from build123d import *

# Parameters (mm, degrees)
SKETCH1_R           = 8.75
BOSS_EXTRUDE1_DEPTH = 15
SKETCH2_R           = 1.9
CUT_EXTRUDE1_DEPTH  = 20
SKETCH3_R           = 1.9
CUT_EXTRUDE2_DEPTH  = 10
SKETCH4_W           = 24.600517232
SKETCH4_H           = 3.517349106
SKETCH4_W_2         = 3.50600932
SKETCH4_W_3         = 2.117023419
CUT_EXTRUDE3_DEPTH  = 129
SKETCH5_W           = 14.928012143
SKETCH5_H           = 3.517349106
CUT_EXTRUDE4_DEPTH  = 39.5


with BuildPart() as part:
    # Sketch1 → Boss-Extrude1 (new body)
    with BuildSketch(Plane(origin=(0, 0, 0), x_dir=(1, 0, 0), z_dir=(0, 1, 0))):
        with BuildLine():
            Line((7.55, -6.557247898), (7.55, -9.961620247))
            Line((7.55, -9.961620247), (14.289149279, -9.92724627))
            Line((14.289149279, -9.92724627), (14.289149279, -7.931016803))
            Line((14.289149279, -7.931016803), (8.967681349, -7.931016803))
            Line((8.967681349, -7.931016803), (8.967681349, -4.425007483))
            ThreePointArc((8.967681349, -4.425007483), (9.738501258, -2.271914007), (10, 0))
            ThreePointArc((10, 0), (-0.861319558, 10.861319558), (-11.722639117, 0))
            Line((-11.722639117, 0), (-11.722639117, -16.005864092))
            Line((-11.722639117, -16.005864092), (-10, -16.005864092))
            Line((-10, -16.005864092), (-10, 0))
            ThreePointArc((-10, 0), (-3.5, -9.367496998), (7.55, -6.557247898))
        make_face()
        with Locations(Location((0, 0, 0), (0, 0, 270))):
            Circle(SKETCH1_R, mode=Mode.SUBTRACT)
    extrude(amount=-BOSS_EXTRUDE1_DEPTH)

    # Sketch2 → Cut-Extrude1 (cut, symmetric)
    with BuildSketch(Plane.ZY.offset(10.823854245)):
        with Locations(Location((12.870484291, -12, 0), (0, 0, 180))):
            Circle(SKETCH2_R)
        with Locations(Location((12.870484291, -3, 0), (0, 0, 180))):
            Circle(SKETCH2_R)
    extrude(amount=CUT_EXTRUDE1_DEPTH, both=True, mode=Mode.SUBTRACT)

    # Sketch3 → Cut-Extrude2 (cut)
    with BuildSketch(Plane(origin=(0, 0, 7.931016803), x_dir=(-1, 0, 0), z_dir=(0, 0, -1))):
        with Locations((-11.586638558, -12.051447382)):
            Circle(SKETCH3_R)
        with Locations((-11.586638558, -3.07185738)):
            Circle(SKETCH3_R)
    extrude(amount=-CUT_EXTRUDE2_DEPTH, mode=Mode.SUBTRACT)

    # Sketch4 → Cut-Extrude3 (cut)
    with BuildSketch(Plane(origin=(8.967681349, 0, 0), x_dir=(0, 0, -1), z_dir=(1, 0, 0))):
        with Locations((7.875251133, -7.5)):
            Rectangle(SKETCH4_W, SKETCH4_H)
        with Locations((-6.178012143, -7.5)):
            Rectangle(SKETCH4_W_2, SKETCH4_H)
        with Locations((-8.989528513, -7.5)):
            Rectangle(SKETCH4_W_3, SKETCH4_H)
    extrude(amount=-CUT_EXTRUDE3_DEPTH, mode=Mode.SUBTRACT)

    # Sketch5 → Cut-Extrude4 (cut, symmetric)
    with BuildSketch(Plane(origin=(-10, 0, 0), x_dir=(0, 0, -1), z_dir=(1, 0, 0))):
        with Locations((1.285993928, -7.5)):
            Rectangle(SKETCH5_W, SKETCH5_H)
    extrude(amount=CUT_EXTRUDE4_DEPTH, both=True, mode=Mode.SUBTRACT)


solid = part.part
Read the model definition and answer for the solid it produces. Units are mm, in the model's axes. A direction names the side the tool comes from. Round coordinates to 2 decimals unless told otherwise and drop trailing zeros. Order: outer loops, then holes, each group sorted by start corner. A loop starts at its lowest first (then second) coordinate and runs counter-clockwise, first axis right, second up. Notation, with made-up numbers: (45, -7) - (60, -7) arc R21 ccw to (60, 11) - close; hole circle Ø7 at (52, 24.25). An arc over 180 degrees is marked (long way). Use one line per item in the form item = value. Start each with the question number.
(1) Flat-ended cylindrical pins translate along their axes: pin 1 Ø3.5 at (y, z) = (-12, 12.87) entering from +X; pin 2 Ø0.9 at (x, y) = (-11, -7.5) entering from -Z; pin 3 Ø6 at (x, y) = (-7.5, -8) entering from -Z; pin 4 Ø2 at (x, y) = (2, -6.5) entering from +Z. Find the tip coordinate at first contact, or state that the pin passes through.
(2) For faces 5 (the face through (7.55, -12, 8)), 6 (the face through (-9, -9.259, 0)), 7 (the face through (12, -7, 7.931)), 8 (the face through (-11, -8, 10.048)), determine the directions among +Z, -Z, +X, -X, +Y, -Y from which every point of the face is accessible in a straight line to the end or side of a thin tool.
(3) Determine the mould class of faces 1 (the face through (8.968, -3, 6)), 2 (the face through (-0.62, -2.83, -10.86)), 3 (the face through (-3.659, -2.83, 9.307)), 4 (the face through (-10.87, -3.08, 14.77)) for opening direction X: +X half, -X half, draft (parallel to the pull), parting line (faces both ways), or undercut.
(4) The part is cut by section A-A (y = -6.5). Give the vertices of the cut face in (x, z), then the cut area to 3 significant figures.
(5) The part is cut by section B-B (y = -1.75). Give the vertices of the cut face in (x, z) (3 decimals).
(6) The part is cut by section C-C (z = -3.5). Give the vertices of the cut face in (x, y), then the cut area to 3 significant figures.
(7) Find the intervals of material crossed by line 1 along Y through (x, z) = (0.5, -9.5); line 2 along X through (y, z) = (-13.25, 6); line 3 along X through (y, z) = (-0.5, 6.75), in increasing order. Write a range as from..to.
(8) The part is cut by section D-D (z = 4.75). Give the vertices of the cut face in (x, y).
Checked values:
q1.pin_1 = through
q1.pin_2 = 10.05
q1.pin_3 = -10.13
q1.pin_4 = 9.91
q2.face_5 = +Z, +Y, -Y
q2.face_6 = -Z, -X
q2.face_7 = +X, +Y, -Y
q2.face_8 = -Z, +X, -X
q3.face_1 = +X half
q3.face_2 = parting line
q3.face_3 = undercut
q3.face_4 = draft
q4.outline = (-11.72, 10.05) - (-10, 10.05) - (-10, 16.01) - (-11.72, 16.01) - close; (8.97, 7.93) - (14.29, 7.93) - (14.29, 9.93) - (8.97, 9.95) - close
q4.area = 21.0 mm^2
q5.outline = (-11.723, 0) arc R10.861 ccw to (10, 0) arc R10 ccw to (8.968, 4.425) - (8.968, 7.931) - (10.222, 7.931) - (10.222, 9.948) - (7.55, 9.962) - (7.55, 6.557) arc R10 ccw to (-10, 0) - (-10, 11.44) - (-11.723, 11.44) - close; (-11.723, 14.301) - (-10, 14.301) - (-10, 16.006) - (-11.723, 16.006) - close; (12.951, 7.931) - (14.289, 7.931) - (14.289, 9.927) - (12.951, 9.934) - close; hole circle Ø17.5 at (0, 0)
q6.outline = (-11.14, -15) - (-8.02, -15) - (-8.02, -9.26) - (-11.14, -9.26) - close; (-11.14, -5.74) - (-8.02, -5.74) - (-8.02, 0) - (-11.14, 0) - close; (8.02, -15) - (9.42, -15) - (9.42, -9.26) - (8.02, -9.26) - close; (8.02, -5.74) - (9.42, -5.74) - (9.42, 0) - (8.02, 0) - close
q6.area = 52.0 mm^2
q7.line_1 = -15..-9.26, -5.74..0
q7.line_2 = -11.72..-10, -8..-6.37, 6.37..8.97
q7.line_3 = -11.72..-10, -7.38..-5.57, 5.57..7.38, 7.55..8.97
q8.outline = (-11.72, -15) - (-10, -15) - (-10, -9.26) - (-11.72, -9.26) - close; (-11.72, -5.74) - (-10, -5.74) - (-10, 0) - (-11.72, 0) - close; (-8.8, -15) - (-7.35, -15) - (-7.35, -9.26) - (-8.8, -9.26) - close; (-8.8, -5.74) - (-7.35, -5.74) - (-7.35, 0) - (-8.8, 0) - close; (7.35, -15) - (8.97, -15) - (8.97, -9.26) - (7.35, -9.26) - close; (7.35, -5.74) - (8.97, -5.74) - (8.97, 0) - (7.35, 0) - close
